from build123d import *

# Parameters (mm, degrees)
SKETCH1_R         = 215
SKETCH1_R_2       = 143
PLATE_DEPTH       = 10
SKETCH2_R         = 204
SKETCH2_R_2       = 144
COMB_GROOVE_DEPTH = 4
SKETCH3_R         = 2.75
ROD_HOLES_DEPTH   = 10


with BuildPart() as part:
    # Sketch1 → Plate (new body)
    with BuildSketch(Plane.XY):
        Circle(SKETCH1_R)
        Circle(SKETCH1_R_2, mode=Mode.SUBTRACT)
    extrude(amount=PLATE_DEPTH)

    # Sketch2 → Comb_groove (cut)
    with BuildSketch(Plane.XY):
        Circle(SKETCH2_R)
        Circle(SKETCH2_R_2, mode=Mode.SUBTRACT)
    extrude(amount=COMB_GROOVE_DEPTH, mode=Mode.SUBTRACT)

    # Sketch3 → Rod_holes (cut)
    with BuildSketch(Plane.XY):
        with Locations((198.770811906, 64.584551824)):
            Circle(SKETCH3_R)
        with Locations((0, 209)):
            Circle(SKETCH3_R)
        with Locations((-198.770811906, 64.584551824)):
            Circle(SKETCH3_R)
        with Locations((-122.847117729, -169.084551824)):
            Circle(SKETCH3_R)
        with Locations((122.847117729, -169.084551824)):
            Circle(SKETCH3_R)
    extrude(amount=ROD_HOLES_DEPTH, mode=Mode.SUBTRACT)


solid = part.part
The model under review builds one solid part; all positions refer to its coordinate system, in mm. A direction names the side the tool comes from. Round coordinates to 2 decimals unless told otherwise and drop trailing zeros. Write each loop counter-clockwise with the first axis right and the second up, starting at its lowest first coordinate (ties: lowest second). Pieces come first, ordered by that corner, then holes. Notation, with made-up numbers: M 8,73.25 L 18,73.25 A30 ccw 18,96.25 Z; hole C 11,61 d1. An arc over 180 degrees is marked long. Use a Markdown table: item, result. Add a question column.
Q1. To check wall thickness, follow line 1 (X direction, y = -3.5, z = 3.5); line 2 (Y direction, x = 0, z = 2.25); line 3 (Y direction, x = 16.5, z = 3). State the ranges of each line that lie inside material, in increasing order.
Q2. The part is to be moulded in two halves that separate along X. For faces 1 (the face through (-44.22, -199.15, 1.97)), 2 (the face through (-105.397, 96.646, 4.93)), 3 (the face through (-170.62, -130.82, 4.93)), 4 (the face through (79, -190, 0)), say which applies: pulls with the +X half, pulls with the -X half, needs draft (parallel to the pull), parting line crosses it, or undercut.
Q3. We need section B-B, the plane z = 2.5. Count the separate pieces of the cut face and the enclosed holes in it, plus the area to 3 significant figures.
Q4. Insertion check: pin 1 (6 mm diameter, centred on y = 110, z = 3.5, fed in from -X); pin 2 (4.5 mm diameter, centred on x = -122.85, y = -169.08, fed in from -Z); pin 3 (4 mm diameter, centred on x = 130.5, z = 2, fed in from -Y); pin 4 (5 mm diameter, centred on x = 37, z = 8, fed in from -Y). Each pin has a flat end and moves straight along its axis. Give the tip position at first contact, or say it passes through.
Q5. Machinability: for faces 5 (the face through (45, -140, 10)), 6 (the face through (-18.746, 142.775, 1.972)), which of the approach directions +Z, -Z, +X, -X, +Y, -Y give a long, thin tool a straight path to every point of the face, cutting with its end or side? Answer none if there is none.
Q6. We need section C-C, the plane x = -133. State the section outline as (y, z) points.
Q7. We need section A-A, the plane y = 0. State the section outline as (x, z) points.
Findings below:
| question | item | result |
|---|---|---|
| 1 | line 1 | x = -214.97 to -203.97, -143.96 to -142.96, 142.96 to 143.96, 203.97 to 214.97 |
| 1 | line 2 | y = -215 to -204, -144 to -143, 143 to 144, 204 to 206.25, 211.75 to 215 |
| 1 | line 3 | y = -214.37 to -203.33, -143.05 to -142.04, 142.04 to 143.05, 203.33 to 214.37 |
| 2 | face 1 | undercut |
| 2 | face 2 | undercut |
| 2 | face 3 | parting line crosses it |
| 2 | face 4 | needs draft |
| 3 | separate pieces | 2 |
| 3 | enclosed holes | 7 |
| 3 | area | 15,300 mm² |
| 4 | pin 1 | stops at x = -186.48 |
| 4 | pin 2 | passes through |
| 4 | pin 3 | stops at y = -172.37 |
| 4 | pin 4 | stops at y = -212.21 |
| 5 | face 5 | +Z, +X, -X, +Y, -Y |
| 5 | face 6 | -Z |
| 6 | outline | M -168.93,0 L -154.68,0 L -154.68,4 L -55.2,4 L -55.2,0 L -52.54,0 L -52.54,10 L -168.93,10 Z; M 52.54,0 L 55.2,0 L 55.2,4 L 154.68,4 L 154.68,0 L 168.93,0 L 168.93,10 L 52.54,10 Z |
| 7 | outline | M -215,0 L -204,0 L -204,4 L -144,4 L -144,0 L -143,0 L -143,10 L -215,10 Z; M 143,0 L 144,0 L 144,4 L 204,4 L 204,0 L 215,0 L 215,10 L 143,10 Z |
